from build123d import *

# Parameters (mm, degrees)
F0_R     = 9.92251
F1_DEPTH = 44.45
F2_W     = 73.0504
F2_H     = 65.0875
F3_DEPTH = 57.151
F4_R     = 10.3251
F5_DEPTH = 7.9375
F6_R     = 12.7
F7_R     = 4.7625


with BuildPart() as f1:
    # F0 (on Front) → F1 (new body, symmetric)
    with BuildSketch(Plane.XZ):
        with BuildLine():
            Line((0, 44.45), (0, 0))
            Line((0, 0), (57.15, 0))
            Line((57.15, 0), (57.15, 44.45))
            ThreePointArc((57.15, 44.45), (28.575, 73.025), (0, 44.45))
        make_face()
        with Locations((28.575, 44.45)):
            Circle(F0_R, mode=Mode.SUBTRACT)
    extrude(amount=F1_DEPTH, both=True)

    # F2 (on Right) → F3 (cut, through all)
    with BuildSketch(Plane.YZ):
        with Locations((0, 40.48125)):
            Rectangle(F2_W, F2_H)
    extrude(amount=F3_DEPTH, mode=Mode.SUBTRACT)

    # F4 (on face) → F5 (join)
    with BuildSketch(Plane.XY.offset(7.9375)):
        with BuildLine():
            ThreePointArc((57.15, -29.063594), (59.009872, -24.573466), (63.5, -22.713594))
            Line((63.5, -22.713594), (111.125, -22.713594))
            ThreePointArc((111.125, -22.713594), (133.304453, -0.488594), (111.125, 21.736406))
            Line((111.125, 21.736406), (63.5, 21.834106))
            ThreePointArc((63.5, 21.834106), (59.009872, 23.693978), (57.15, 28.184106))
            Line((57.15, 28.184106), (57.15, -29.063594))
        make_face()
        with Locations((73.025, -0.149807)):
            Circle(F4_R, mode=Mode.SUBTRACT)
        with Locations((111.125, -0.227967)):
            Circle(F4_R, mode=Mode.SUBTRACT)
    extrude(amount=-F5_DEPTH)

    # F6
    f6_edges = [f1.edges().sort_by_distance(p)[0] for p in [
        (28.575, -44.45, 0),
        (28.575, 44.45, 0),
    ]]
    fillet(f6_edges, radius=F6_R)

    # F7
    f7_edges = [f1.edges().sort_by_distance(p)[0] for p in [
        (28.575, -36.5252, 7.9375),
        (28.575, 36.5252, 7.9375),
    ]]
    fillet(f7_edges, radius=F7_R)


solid = f1.part
The model under review builds one solid part; all positions refer to its coordinate system, in mm. A direction names the side the tool comes from. Round coordinates to 2 decimals unless told otherwise and drop trailing zeros. Write each loop counter-clockwise with the first axis right and the second up, starting at its lowest first coordinate (ties: lowest second). Pieces come first, ordered by that corner, then holes. Notation, with made-up numbers: M -39,32 L 12,32 A26 cw 12,70 Z; hole C 32,-1.5 d5. An arc over 180 degrees is marked long. Use a Markdown table: item, result. Add a question column.
Q1. The part is to be moulded in two halves that separate along X. For faces 1 (the face through (22, -36.525, 36)), 2 (the face through (59.06, 23.645, 4.024)), 3 (the face through (0, -0.6, 7.7)), 4 (the face through (26.424, -40.432, 34.763)), say which applies: pulls with the +X half, pulls with the -X half, needs draft (parallel to the pull), parting line crosses it, or undercut.
Q2. To check wall thickness, follow line 1 (Y direction, x = 46, z = 22); line 2 (X direction, y = -42, z = 44.45); line 3 (Z direction, x = 33, y = 28). State the ranges of each line that lie inside material, in increasing order.
Q3. We need section D-D, the plane y = 26. State the section outline as (x, z) points.
Q4. Machinability: for faces 5 (the face through (87, -22.714, 4)), 6 (the face through (29, 35.1, 9.3)), 7 (the face through (57.15, 38, 22)), 8 (the face through (29.2, 40.43, 73.02)), which of the approach directions +Z, -Z, +X, -X, +Y, -Y give a long, thin tool a straight path to every point of the face, cutting with its end or side? Answer none if there is none.
Q5. Insertion check: pin 1 (10 mm diameter, centred on x = 96, y = -26, fed in from +Z); pin 2 (6.5 mm diameter, centred on x = 94, z = 5.5, fed in from -Y); pin 3 (12.5 mm diameter, centred on y = -36.5, z = 19, fed in from +X). Each pin has a flat end and moves straight along its axis. Give the tip position at first contact, or say it passes through.
Q6. We need section B-B, the plane z = 48. State the section outline as (x, y) points, plus the area to 3 significant figures.
Q7. We need section A-A, the plane z = 23. State the section outline as (x, y) points.
Findings below:
| question | item | result |
|---|---|---|
| 1 | face 1 | needs draft |
| 1 | face 2 | pulls with the +X half |
| 1 | face 3 | pulls with the -X half |
| 1 | face 4 | undercut |
| 2 | line 1 | y = -44.45 to -36.53, 36.53 to 44.45 |
| 2 | line 2 | x = 0 to 18.65, 38.5 to 57.15 |
| 2 | line 3 | z = 0 to 7.94 |
| 3 | outline | M 0,0 L 57.54,0 L 57.54,7.94 L 0,7.94 Z |
| 4 | face 5 | +Z, -Z, +X, -Y |
| 4 | face 6 | +Z, +X, -X |
| 4 | face 7 | +Z, -Z, +X, +Y |
| 4 | face 8 | +Z, +Y, -Y |
| 5 | pin 1 | stops at z = 7.94 |
| 5 | pin 2 | stops at y = -22.71 |
| 5 | pin 3 | stops at x = 57.15 |
| 6 | outline | M 0.22,-44.45 L 19.31,-44.45 L 19.31,-36.53 L 0.22,-36.53 Z; M 0.22,36.53 L 19.31,36.53 L 19.31,44.45 L 0.22,44.45 Z; M 37.84,-44.45 L 56.93,-44.45 L 56.93,-36.53 L 37.84,-36.53 Z; M 37.84,36.53 L 56.93,36.53 L 56.93,44.45 L 37.84,44.45 Z |
| 6 | area | 605 mm² |
| 7 | outline | M 0,-44.45 L 57.15,-44.45 L 57.15,-36.53 L 0,-36.53 Z; M 0,36.53 L 57.15,36.53 L 57.15,44.45 L 0,44.45 Z |
